Autodesk Inventor part; units mm, degrees
ref_plane "YZ Plane" through (0, 0, 0) normal (1, 0, 0) x (0, 1, 0)
ref_plane "XZ Plane" through (0, 0, 0) normal (0, 1, 0) x (-1, 0, 0)
ref_plane "XY Plane" through (0, 0, 0) normal (0, 0, 1) x (1, 0, 0)
sketch "Sketch1" plane through (0, 0, 0) normal (1, 0, 0) x (0, 1, 0)
  line L0 (3.556, -2.0531) -> (0, -4.1061)
  line L1 (0, -4.1061) -> (-3.556, -2.0531)
  line L2 (-3.556, -2.0531) -> (-3.556, 2.0531)
  line L3 (-3.556, 2.0531) -> (0, 4.1061)
  line L4 (0, 4.1061) -> (3.556, 2.0531)
  line L5 (3.556, 2.0531) -> (3.556, -2.0531)
  point P0 (0, 0)
  point P1 (0, 0)
  dimension "d0" = 7.112
extrude "Extrusion1" add sketch "Sketch1" along normal blind 3.429
sketch "Sketch2" plane through (0, 0, 0) normal (-1, 0, 0) x (0, 0, 1)
  circle A0 centre (0, 0) radius 3.4036
  dimension "d3" = 6.8072
extrude "Extrusion2" add sketch "Sketch2" along normal blind 3.175
sketch "Sketch3" plane through (-3.175, 0, 0) normal (-1, 0, 0) x (0, 0, 1)
  circle A0 centre (0, 0) radius 3.4036
hole "Hole1" at (-3.175, 0, 0) direction (1, 0, 0) diameter 5.334 end through all
thread "Thread1"
properties part number "Hex Cap"
Can you work these out from the model? Positions are in its coordinate system, mm. A direction names the side the tool comes from. Round coordinates to 2 decimals unless told otherwise and drop trailing zeros. Loops run counter-clockwise (first coordinate to the right, second up) from the corner with the lowest first, then second, coordinate; pieces in that order, holes last. Notation, with made-up numbers: (87.25, 25) -> (94.25, 25) arc R23 ccw to (94.25, 64) -> close; hole circle Ø7 at (39, 45). An arc over 180 degrees is marked (long way). One line per item, written item: value. Start each with the question number.
1. If we mould it in two halves opening along Z, with no side actions, what happens to faces 3 (the flat face through (1.69, -1.753, -3.094)), 4 (the cylindrical face through (0.173, 2.366, 1.231)), 5 (the flat face through (1.69, 1.753, 3.094)), 6 (the flat face through (-3.175, -2, -2))? For each: pulls with the +Z half, pulls with the -Z half, needs draft (parallel to the pull), parting line crosses it, or undercut.
2. If we section it at D-D, the plane z = 3: Write out the boundary of the cut face in (x, y) (3 decimals).
3. For faces 1 (the flat face through (2, 3.556, 0)), 2 (the cylindrical face through (-1.565, 1.304, 3.144)), which set-ups out of +Z, -Z, +X, -X, +Y, -Y let a thin tool reach every point of the face, with its end or its side?
4. If we section it at A-A, the plane z = 0: Write out the boundary of the cut face in (x, y) (3 decimals).
5. If we section it at B-B, the plane x = 1.75: Write out the boundary of the cut face in (y, z).
6. If we section it at C-C, the plane y = 0.5: Write out the boundary of the cut face in (x, z) (3 decimals).
7. If I drill on probe 1 along Y at (x, z) = (-0.5, 0); probe 2 along Y at (x, z) = (0.5, 0); probe 3 along Z at (x, y) = (-2.5, 2.25), over which ranges is the centre line in solid material (lowest first)?
Calculated:
1. face 3: pulls with the -Z half
1. face 4: undercut
1. face 5: pulls with the +Z half
1. face 6: needs draft
2. outline: (-3.175, -1.608) -> (0, -1.608) -> (0, -1.916) -> (3.429, -1.916) -> (3.429, 1.916) -> (0, 1.916) -> (0, 1.608) -> (-3.175, 1.608) -> close
3. face 1: +Z, -Z, +X, -X, +Y
3. face 2: -X
4. outline: (-3.175, -3.404) -> (0, -3.404) -> (0, -3.556) -> (3.429, -3.556) -> (3.429, -2.667) -> (-3.175, -2.667) -> close; (-3.175, 2.667) -> (3.429, 2.667) -> (3.429, 3.556) -> (0, 3.556) -> (0, 3.404) -> (-3.175, 3.404) -> close
5. outline: (-3.56, -2.05) -> (0, -4.11) -> (3.56, -2.05) -> (3.56, 2.05) -> (0, 4.11) -> (-3.56, 2.05) -> close; hole circle Ø5.33 at (0, 0)
6. outline: (-3.175, -3.367) -> (0, -3.367) -> (0, -3.817) -> (3.429, -3.817) -> (3.429, -2.62) -> (-3.175, -2.62) -> close; (-3.175, 2.62) -> (3.429, 2.62) -> (3.429, 3.817) -> (0, 3.817) -> (0, 3.367) -> (-3.175, 3.367) -> close
7. probe 1: y = -3.4 to -2.67, 2.67 to 3.4
7. probe 2: y = -3.56 to -2.67, 2.67 to 3.56
7. probe 3: z = -2.55 to -1.43, 1.43 to 2.55
